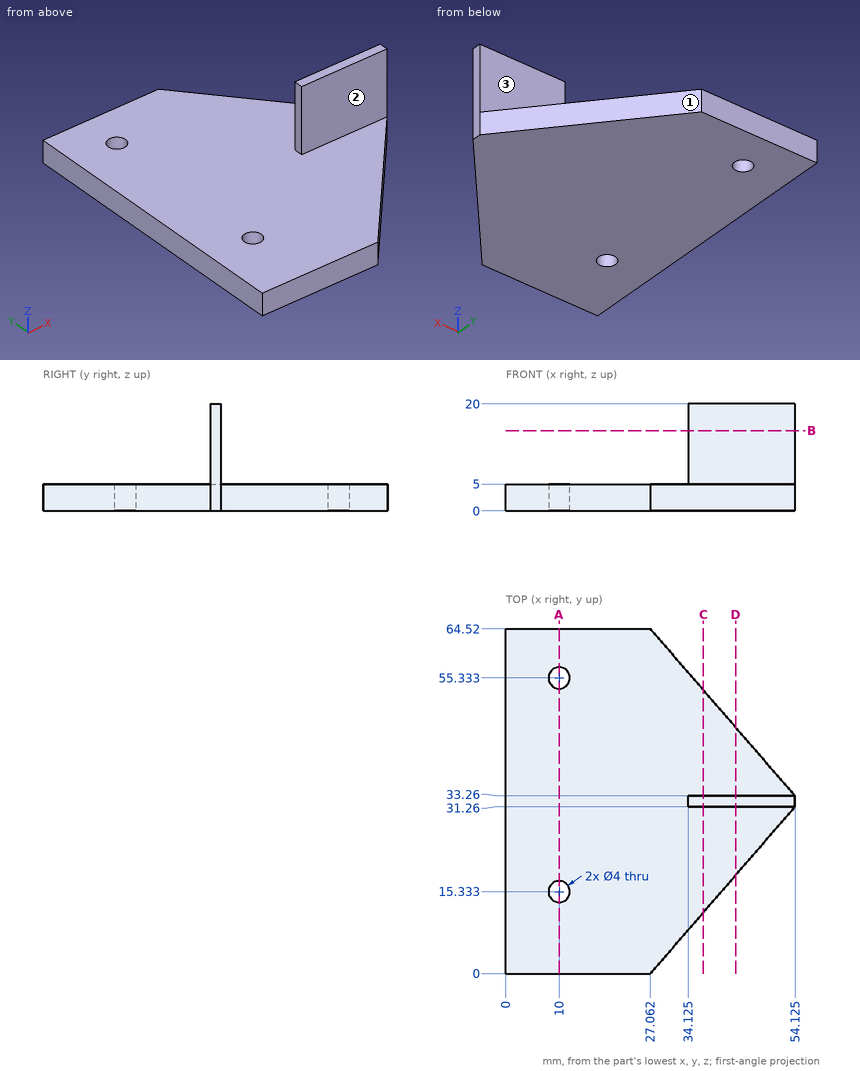
Can you work these out from the drawing? Everything is in mm from the part's minimum corner. A direction names the side the tool comes from. Coordinates: 2 decimals unless noted, no trailing zeros. Loops run counter-clockwise (first coordinate to the right, second up) from the corner with the lowest first, then second, coordinate; pieces in that order, holes last.
1) Imagine slicing it at B-B on z = 15. List the corners of the cut face in (x, y) for me (1 decimal), plus the area to 3 significant figures.
2) I need wall thicknesses on probe 1 along Y at (x, z) = (10, 2.65); probe 2 along Z at (x, y) = (33, 17); probe 3 along Y at (x, z) = (36, 15.5). Which ranges of each line are inside material? Lowest first, please.
3) Imagine slicing it at C-C on x = 37. List the corners of the cut face in (y, z) for me.
4) Imagine slicing it at A-A on x = 10. List the corners of the cut face in (y, z) for me.
5) For pin 1 (7.5 mm diameter, centred on x = 44.5, z = 13, fed in from +Y); pin 2 (6 mm diameter, centred on x = 20, z = 5.5, fed in from -Y); pin 3 (5 mm diameter, centred on x = 42.5, z = 8, fed in from -Y); pin 4 (10 mm diameter, centred on x = 7, y = 33.5, fed in from +Z), each with a flat end and sliding along its axis, tell me the tip position at first contact or that it passes through.
6) Imagine slicing it at D-D on x = 43. List the corners of the cut face in (y, z) for me.
7) Which directions (+Z, -Z, +X, -X, +Y, -Y) give clear straight access to the entire face, cutting with the end or side of a thin tool? Please do the marked faces 1, 2 and 3.
Completed:
1. outline: (34.1, 31.3) - (54.1, 31.3) - (54.1, 33.3) - (34.1, 33.3) - close
1. area: 40.0 mm2
2. probe 1: y = 0 to 13.33, 17.33 to 53.33, 57.33 to 64.52
2. probe 2: z = 0 to 5
2. probe 3: y = 31.26 to 33.26
3. outline: (11.48, 0) - (53.04, 0) - (53.04, 5) - (33.26, 5) - (33.26, 20) - (31.26, 20) - (31.26, 5) - (11.48, 5) - close
4. outline: (0, 0) - (13.33, 0) - (13.33, 5) - (0, 5) - close; (17.33, 0) - (53.33, 0) - (53.33, 5) - (17.33, 5) - close; (57.33, 0) - (64.52, 0) - (64.52, 5) - (57.33, 5) - close
5. pin 1: stops at y = 33.26
5. pin 2: stops at y = 0
5. pin 3: stops at y = 31.26
5. pin 4: stops at z = 5
6. outline: (18.41, 0) - (46.11, 0) - (46.11, 5) - (33.26, 5) - (33.26, 20) - (31.26, 20) - (31.26, 5) - (18.41, 5) - close
7. face 1: +Z, -Z, +X, +Y
7. face 2: +Z, +X, -X, -Y
7. face 3: +Z, +X, -X, +Y
